The model under review builds one solid part; all positions refer to its coordinate system, in mm. A direction names the side the tool comes from. Coordinates: 2 decimals unless noted, no trailing zeros. Write each loop counter-clockwise with the first axis right and the second up, starting at its lowest first coordinate (ties: lowest second). Pieces come first, ordered by that corner, then holes. Notation, with made-up numbers: (38, 69.5) - (93, 69.5) arc R11 ccw to (93, 73.5) - close; hole circle Ø10 at (21, 25.25). An arc over 180 degrees is marked (long way). Return JSON: item names as keys, results as strings. Group by question number.
(1) We need section C-C on x = 0. State the section outline as (y, z) points (1 decimal).
(2) We need section D-D on y = 50.8. State the section outline as (x, z) points (3 decimals).
(3) We need section A-A on z = 0. State the section outline as (x, y) points (1 decimal).
(4) For pin 1 Ø6 at (x, y) = (0, 50.8) entering from -Z; pin 2 Ø5.5 at (x, y) = (0, 53) entering from +Z, all flat-tipped, find the tip position at first contact; note any pin that passes through.
(5) To check wall thickness, follow L1, parallel to Y at x = 0, z = 9.25; L2, parallel to Y at x = 0.25, z = 0; L3, parallel to Y at x = 0, z = -9.25. State the ranges of each line that lie inside material, in increasing order. Write a range as from..to.
(6) Draft analysis for pull direction Z (two halves, no side actions). For faces 1 (the face through (0, 88.646, 0)), 2 (the face through (4, 51, 3.048)), 3 (the face through (0.12, 71.48, 0.62)), 4 (the face through (0, 41, -12.7)), state which applies: released by +Z, released by -Z, zero draft, split by the parting line, or undercut.
(7) Tool access review of faces 5 (the face through (5.3, 1.67, 7.94)), 6 (the face through (-9.525, 39, 0)): name each direction out of +Z, -Z, +X, -X, +Y, -Y from which nothing blocks a thin tool from reaching the whole face with its end or side.
(8) We need section B-B on y = 76.2. State the section outline as (x, z) points (1 decimal), then the cut area to 3 significant figures.
```python
from build123d import *

# Parameters (mm, degrees)
BOSS_EXTRUDE1_DEPTH                              = 12.7
CBORE_FOR_1_4_SOCKET_HEAD_CAP_SCREW1_D           = 6.7564
CBORE_FOR_1_4_SOCKET_HEAD_CAP_SCREW1_DEPTH       = 25.4
CBORE_FOR_1_4_SOCKET_HEAD_CAP_SCREW1_CBORE_D     = 11.1125
CBORE_FOR_1_4_SOCKET_HEAD_CAP_SCREW1_CBORE_DEPTH = 9.652


with BuildPart() as part:
    # Sketch6 → Boss-Extrude1 (new body, symmetric)
    with BuildSketch(Plane.XY):
        Polygon((-8.001, 88.646), (8.001, 88.646), (9.525, 87.122), (9.525, -7.366), (8.001, -8.89), (-8.001, -8.89), (-9.525, -7.366), (-9.525, 87.122), align=None)
    extrude(amount=BOSS_EXTRUDE1_DEPTH, both=True)

    # Sketch11 → 3/8-16 Tapped Hole1 (revolve, cut)
    with BuildSketch(Plane(origin=(9.525, 76.2, 0), x_dir=(0, 0, -1), z_dir=(0, 1, 0))):
        Polygon((0, 0), (0, 19.05), (5.3975, 19.05), (4.7625, 18.415), (4.7625, 0.635), (5.3975, 0), align=None)
    revolve(axis=Axis((15.875, 76.2, 0), (-1, 0, 0)), mode=Mode.SUBTRACT)

    # CBORE for 1/4 Socket Head Cap Screw1
    with Locations(Plane.XY.offset(12.7)):
        with Locations((0, 0), (0, 50.8)):
            CounterBoreHole(CBORE_FOR_1_4_SOCKET_HEAD_CAP_SCREW1_D / 2, CBORE_FOR_1_4_SOCKET_HEAD_CAP_SCREW1_CBORE_D / 2, CBORE_FOR_1_4_SOCKET_HEAD_CAP_SCREW1_CBORE_DEPTH, depth=CBORE_FOR_1_4_SOCKET_HEAD_CAP_SCREW1_DEPTH)


solid = part.part
```
Ans:
{
 "1": {"outline": "(-8.9, -12.7) - (-3.4, -12.7) - (-3.4, 3) - (-5.6, 3) - (-5.6, 12.7) - (-8.9, 12.7) - close; (3.4, -12.7) - (47.4, -12.7) - (47.4, 3) - (45.2, 3) - (45.2, 12.7) - (5.6, 12.7) - (5.6, 3) - (3.4, 3) - close; (54.2, -12.7) - (88.6, -12.7) - (88.6, 12.7) - (56.4, 12.7) - (56.4, 3) - (54.2, 3) - close; hole circle Ø9.5 at (76.2, 0)"},
 "2": {"outline": "(-9.525, -12.7) - (-3.378, -12.7) - (-3.378, 3.048) - (-5.556, 3.048) - (-5.556, 12.7) - (-9.525, 12.7) - close; (3.378, -12.7) - (9.525, -12.7) - (9.525, 12.7) - (5.556, 12.7) - (5.556, 3.048) - (3.378, 3.048) - close"},
 "3": {"outline": "(-9.5, -7.4) - (-8, -8.9) - (8, -8.9) - (9.5, -7.4) - (9.5, 70.8) - (8.9, 71.4) - (-8.9, 71.4) - (-9.5, 70.8) - close; (-9.5, 81.6) - (-8.9, 81) - (8.9, 81) - (9.5, 81.6) - (9.5, 87.1) - (8, 88.6) - (-8, 88.6) - (-9.5, 87.1) - close; hole circle Ø6.8 at (0, 0); hole circle Ø6.8 at (0, 50.8)"},
 "4": {"pin 1": "through", "pin 2": "z = 3.05"},
 "5": {"L1": "-8.89..-5.56, 5.56..45.24, 56.36..88.65", "L2": "-8.89..-3.37, 3.37..47.43, 54.17..71.44, 80.96..88.65", "L3": "-8.89..-3.38, 3.38..47.42, 54.18..88.65"},
 "6": {"face 1": "zero draft", "face 2": "released by +Z", "face 3": "undercut", "face 4": "released by -Z"},
 "7": {"face 5": "+Z", "face 6": "+Z, -Z, -X, +Y, -Y"},
 "8": {"outline": "(-9.5, -12.7) - (9.5, -12.7) - (9.5, -5.4) - (8.9, -4.8) - (-8.9, -4.8) - (-9.5, -5.4) - close; (-9.5, 5.4) - (-8.9, 4.8) - (8.9, 4.8) - (9.5, 5.4) - (9.5, 12.7) - (-9.5, 12.7) - close", "area": "302 mm²"}
}
